CAD build for the part. Positions are in the model's coordinates, mm. A direction names the side the tool comes from. Give positions to 0.01 mm unless a question says otherwise; leave off trailing zeros. Write each loop counter-clockwise with the first axis right and the second up, starting at its lowest first coordinate (ties: lowest second). Pieces come first, ordered by that corner, then holes. Notation, with made-up numbers: (21, 6.25) -> (26, 6.25) arc R18 cw to (26, 18.25) -> close; hole circle Ø8 at (13, 15). An arc over 180 degrees is marked (long way). Answer as a JSON object with one key per item and string values.
```python
from build123d import *

# Parameters (mm, degrees)
F0_W     = 7
F0_H     = 6
F1_DEPTH = 12.5
F2_R     = 3
F2_R_2   = 1.8
F3_DEPTH = 2.5
F4_W     = 0.5
F4_H     = 1
F5_DEPTH = 1.3


with BuildPart() as f1:
    # F0 (on Front) → F1 (new body)
    with BuildSketch(Plane.XZ):
        with Locations((3.5, 3)):
            Rectangle(F0_W, F0_H)
    extrude(amount=F1_DEPTH)

    # F2 (on face) → F3 (join)
    with BuildSketch(Plane.XZ.offset(12.5)):
        with Locations((3.5, 3)):
            Circle(F2_R)
        with Locations((3.5, 3)):
            Circle(F2_R_2, mode=Mode.SUBTRACT)
    extrude(amount=F3_DEPTH)

    # F4 (on face) → F5 (join)
    with BuildSketch(Plane(origin=(0, 0, 0), x_dir=(1, 0, 0), z_dir=(0, 0, -1))):
        with Locations((0.25, 0.5)):
            Rectangle(F4_W, F4_H)
        with Locations((0.25, 10.5)):
            Rectangle(F4_W, F4_H)
        with Locations((6.75, 10.5)):
            Rectangle(F4_W, F4_H)
        with Locations((6.75, 0.5)):
            Rectangle(F4_W, F4_H)
    extrude(amount=F5_DEPTH)


solid = f1.part
```
1) Slice it at C-C (y = -5.5). List the corners of the cut face in (x, z), then the cut area to 3 significant figures.
Model answer:
{"outline": "(0, 0) -> (7, 0) -> (7, 6) -> (0, 6) -> close", "area": "42.0 mm2"}
2) Slice it at A-A (z = 3). List the corners of the cut face in (x, y).
Model answer:
{"outline": "(0, -12.5) -> (0.5, -12.5) -> (0.5, -15) -> (1.7, -15) -> (1.7, -12.5) -> (5.3, -12.5) -> (5.3, -15) -> (6.5, -15) -> (6.5, -12.5) -> (7, -12.5) -> (7, 0) -> (0, 0) -> close"}
3) Mould opens along Y. For faces 1 (the flat face through (6.7, -12.5, 3.2)), 2 (the flat face through (0.5, -10.5, -0.6)), 3 (the flat face through (3, 0, 3)), 4 (the flat face through (3, -6, 0)) say: released by +Y, released by -Y, zero draft, split by the parting line, or undercut.
Model answer:
{"face 1": "released by -Y", "face 2": "zero draft", "face 3": "released by +Y", "face 4": "undercut"}
4) Wall check: probe 1 along Z at (x, y) = (3.5, -14.45); probe 2 along Y at (x, z) = (0.75, 1.25); probe 3 along Z at (x, y) = (6.75, -3.5). Give the ranges that are in metal, low to high.
Model answer:
{"probe 1": "z = 0 to 1.2, 4.8 to 6", "probe 2": "y = -12.5 to 0", "probe 3": "z = 0 to 6"}
5) 3-axis set-ups, long thin cutter, end or side, ignore diameter. For faces 5 (the flat face through (0, -6, 3)), 6 (the flat face through (0.3, -12.5, 3.5)), 7 (the cylindrical face through (1.29, -13.73, 5.03)), 8 (the flat face through (3, -6, 6)), 9 (the flat face through (6.5, -0.5, -0.6)): which of +Z, -Z, +X, -X, +Y, -Y reach the whole face in a straight line?
Model answer:
{"face 5": "+Z, -Z, -X, +Y, -Y", "face 6": "-X, -Y", "face 7": "-Y", "face 8": "+Z, +X, -X, +Y, -Y", "face 9": "-Z, +Y, -Y"}
6) Slice it at D-D (z = 5.5). List the corners of the cut face in (x, y).
Model answer:
{"outline": "(0, -12.5) -> (1.84, -12.5) -> (1.84, -15) -> (5.16, -15) -> (5.16, -12.5) -> (7, -12.5) -> (7, 0) -> (0, 0) -> close"}
7) Pin check, flat tips, straight feed: pin 1 (0.6 mm diameter, centred on x = 0.5, z = -0.5, fed in from -Y); pin 2 (3 mm diameter, centred on x = 3.5, z = 3, fed in from -Y). Stop position of each tip, or through.
Model answer:
{"pin 1": "stops at y = -11", "pin 2": "stops at y = -12.5"}
